Verification items for the finished model (mm, model axes). A direction names the side the tool comes from. Coordinates: 2 decimals unless noted, no trailing zeros. Order: outer loops, then holes, each group sorted by start corner. A loop starts at its lowest first (then second) coordinate and runs counter-clockwise, first axis right, second up.
Q1. Cross-section at C-C, the plane y = -38. Record the boundary of the cut face in (x, z), and give its area (3 significant figures).
Q2. Cross-section at A-A, the plane x = 5. Record the boundary of the cut face in (y, z), and give its area (3 significant figures).
Q3. Cross-section at B-B, the plane z = 2. Record the boundary of the cut face in (x, y).
Q4. Cross-section at D-D, the plane x = 19. Record the boundary of the cut face in (y, z).
Q5. Set-up check for faces 4 (the flat face through (12, -15, 12)), 5 (the flat face through (42, 55, 5)), 6 (the flat face through (0, -65, 5)), 7 (the flat face through (12, 70.5, 5)), 8 (the flat face through (17.5, -25, 12)): record each of +Z, -Z, +X, -X, +Y, -Y from which the full face is reachable in a straight line by a thin tool's end or side.
Q6. Draft check along Z on faces 1 (the flat face through (42, -35, 3.5)), 2 (the flat face through (10.25, -70, 5)), 3 (the flat face through (22.5, 65, 5)). Enter one of: pulls with the +Z half, pulls with the -Z half, needs draft (parallel to the pull), parting line crosses it, or undercut.
Q7. Thickness scan on line 1 (X direction, y = 68, z = 3.75); line 2 (Z direction, x = -23.5, y = 32); line 3 (X direction, y = -37, z = 2.5). Record the ranges inside material, lowest first.
Q8. Depth check by flat-ended pin: P1, Ø5, axis at x = 2, y = 15.5, coming from the +Z side; P2, Ø4.5, axis at y = -20.5, z = 11.5, coming from the +X side; P3, Ø3.5, axis at x = 43, z = 4.5, coming from the -Y side. Enter the tip coordinate at first touch or a pass-through.
from build123d import *

# Parameters (mm, degrees)
SKETCH1_W           = 150
SKETCH1_H           = 75
SKETCH1_W_2         = 11
SKETCH1_H_2         = 22
BOSS_EXTRUDE1_DEPTH = 10
SKETCH2_W           = 10
SKETCH2_H           = 20
BOSS_EXTRUDE2_DEPTH = 4
SKETCH3_W           = 20
SKETCH3_H           = 3
BOSS_EXTRUDE3_DEPTH = 10
SKETCH4_W           = 20.5
SKETCH4_H           = 3.2
CUT_EXTRUDE1_DEPTH  = 10


with BuildPart() as part:
    # Sketch1 → Boss-Extrude1 (new body)
    with BuildSketch(Plane(origin=(0, 0, 0), x_dir=(0, 1, 0), z_dir=(0, 0, 1))):
        Rectangle(SKETCH1_W, SKETCH1_H)
        with Locations((65, -11.5)):
            Rectangle(SKETCH1_W_2, SKETCH1_H_2, mode=Mode.SUBTRACT)
    extrude(amount=BOSS_EXTRUDE1_DEPTH)

    # Sketch2 → Boss-Extrude2 (add)
    with BuildSketch(Plane.XY.offset(10)):
        with Locations((12.5, -25)):
            Rectangle(SKETCH2_W, SKETCH2_H)
    extrude(amount=BOSS_EXTRUDE2_DEPTH)

    # Sketch3 → Boss-Extrude3 (add)
    with BuildSketch(Plane.YZ.offset(37.5)):
        with Locations((45, 5)):
            Rectangle(SKETCH3_W, SKETCH3_H)
        with Locations((-35, 5)):
            Rectangle(SKETCH3_W, SKETCH3_H)
    extrude(amount=BOSS_EXTRUDE3_DEPTH)

    # Sketch4 → Cut-Extrude1 (cut)
    with BuildSketch(Plane.XZ.offset(75)):
        with Locations((0, 5)):
            Rectangle(SKETCH4_W, SKETCH4_H)
    extrude(amount=-CUT_EXTRUDE1_DEPTH, mode=Mode.SUBTRACT)


solid = part.part
Check values:
1. outline: (-37.5, 0) - (37.5, 0) - (37.5, 3.5) - (47.5, 3.5) - (47.5, 6.5) - (37.5, 6.5) - (37.5, 10) - (-37.5, 10) - close
1. area: 780 mm2
2. outline: (-75, 0) - (59.5, 0) - (59.5, 10) - (-75, 10) - (-75, 6.6) - (-65, 6.6) - (-65, 3.4) - (-75, 3.4) - close; (70.5, 0) - (75, 0) - (75, 10) - (70.5, 10) - close
2. area: 1,360 mm2
3. outline: (-37.5, -75) - (37.5, -75) - (37.5, 75) - (-37.5, 75) - close; hole (0.5, 59.5) - (22.5, 59.5) - (22.5, 70.5) - (0.5, 70.5) - close
4. outline: (-75, 0) - (59.5, 0) - (59.5, 10) - (-75, 10) - close; (70.5, 0) - (75, 0) - (75, 10) - (70.5, 10) - close
5. face 4: +Z, +X, -X, +Y
5. face 5: +Z, -Z, +X, +Y
5. face 6: -Y
5. face 7: +Z, -Z
5. face 8: +Z, +X, +Y, -Y
6. face 1: pulls with the -Z half
6. face 2: undercut
6. face 3: needs draft
7. line 1: x = -37.5 to 0.5, 22.5 to 37.5
7. line 2: z = 0 to 10
7. line 3: x = -37.5 to 37.5
8. P1: stops at z = 10
8. P2: stops at x = 37.5
8. P3: stops at y = -45
